CAD build for the part. Positions are in the model's coordinates, mm. Face numbers are marked on the shaded views. A direction names the side the tool comes from. Round coordinates to 2 decimals unless told otherwise and drop trailing zeros. Loops run counter-clockwise (first coordinate to the right, second up) from the corner with the lowest first, then second, coordinate; pieces in that order, holes last.
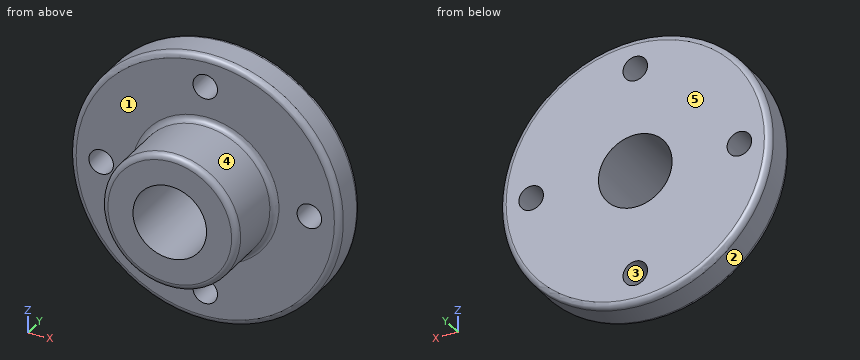
```python
from build123d import *

# Parameters (mm, degrees)
F2_R            = 3.048
F3_R            = 6.35
F4_DEPTH        = 19.051
F4_COPIES_COUNT = 4


# Not quite as in the source:
# - a pattern or mirror of a feature is missing from the dataset's text; its kind, count and spacing are read off the source's solid


with BuildPart() as f1:
    # F0 (on Right) → F1 (revolve)
    with BuildSketch(Plane.YZ):
        Polygon((-53.848, 19.05), (0, 19.05), (0, 69.85), (-19.05, 69.85), (-19.05, 35.052), (-53.848, 35.052), align=None)
    revolve(axis=Axis((0, -30.1634762436, 0), (0, -1, 0)))

    # F2
    f2_edges = [f1.edges().sort_by_distance(p)[0] for p in [
        (0, -53.848, -35.052),
        (0, -19.05, -35.052),
        (0, -19.05, -69.85),
        (0, 0, -69.85),
    ]]
    fillet(f2_edges, radius=F2_R)

    # F3 (on face) → F4 (cut, through all)
    with BuildSketch(Plane.XZ.offset(19.05)):
        with Locations((0, 53.848)):
            Circle(F3_R)
    f4 = extrude(amount=-F4_DEPTH, mode=Mode.SUBTRACT)

    # F4_copies: F4 ×4 about axis
    f4_copies_axis = Axis((0, 0, 0), (0, 1, 0))
    for i in range(1, F4_COPIES_COUNT):
        add(f4.rotate(f4_copies_axis, i * 360 / F4_COPIES_COUNT), mode=Mode.SUBTRACT)


solid = f1.part
```
Item 1: Flat gauge pins, fed straight in: P1, Ø4, axis at x = -24, y = -42.5, coming from the +Z side; P2, Ø6, axis at x = 13.5, y = -29, coming from the -Z side; P3, Ø14.5, axis at x = 0, z = -53.848, coming from the -Y side. Where does each tip first touch, or does it go through?
Answers follow:
P1: stops at z = 27.29
P2: stops at z = -33.44
P3: stops at y = -19.05
Item 2: Cut at D-D, the plane y = -9. Give the cut face in (x, z), plus the area to 3 significant figures.
Answers follow:
outline: circle Ø139.7 at (0, 0); hole circle Ø12.7 at (-53.85, 0); hole circle Ø38.1 at (0, 0); hole circle Ø12.7 at (0, -53.85); hole circle Ø12.7 at (0, 53.85); hole circle Ø12.7 at (53.85, 0)
area: 13,700 mm2
Item 3: Cut at C-C, the plane y = -34.5. Give the cut face in (x, z).
Answers follow:
outline: circle Ø70.1 at (0, 0); hole circle Ø38.1 at (0, 0)
Item 4: 3-axis set-ups, long thin cutter, end or side, ignore diameter. For the marked faces 1 and 2: which of +Z, -Z, +X, -X, +Y, -Y reach the whole face in a straight line?
Answers follow:
face 1: -Y
face 2: +Y, -Y
Item 5: Two-plate mould, pull along Z, no slides. Class the marked faces 3, 4 and 5: released by +Z, released by -Z, zero draft, split by the parting line, or undercut.
Answers follow:
face 3: undercut
face 4: split by the parting line
face 5: zero draft
Item 6: Probe line 1 (Z direction, x = 0, y = -7); line 2 (X direction, y = -34.5, z = 0). List the from-to ranges inside material, lowest first.
Answers follow:
line 1: z = -69.85 to -60.2, -47.5 to -19.05, 19.05 to 47.5, 60.2 to 69.85
line 2: x = -35.05 to -19.05, 19.05 to 35.05
Item 7: Cut at B-B, the plane z = 0. Give the cut face in (x, y), plus the area to 3 significant figures.
Answers follow:
outline: (-69.85, -16) arc R3.05 ccw to (-66.8, -19.05) - (-60.2, -19.05) - (-60.2, 0) - (-66.8, 0) arc R3.05 ccw to (-69.85, -3.05) - close; (-47.5, -19.05) - (-38.1, -19.05) arc R3.05 cw to (-35.05, -22.1) - (-35.05, -50.8) arc R3.05 ccw to (-32, -53.85) - (-19.05, -53.85) - (-19.05, 0) - (-47.5, 0) - close; (19.05, -53.85) - (32, -53.85) arc R3.05 ccw to (35.05, -50.8) - (35.05, -22.1) arc R3.05 cw to (38.1, -19.05) - (47.5, -19.05) - (47.5, 0) - (19.05, 0) - close; (60.2, -19.05) - (66.8, -19.05) arc R3.05 ccw to (69.85, -16) - (69.85, -3.05) arc R3.05 ccw to (66.8, 0) - (60.2, 0) - close
area: 2,560 mm2
Item 8: Cut at A-A, the plane x = 0. Give the cut face in (y, z).
Answers follow:
outline: (-53.85, -32) arc R3.05 ccw to (-50.8, -35.05) - (-22.1, -35.05) arc R3.05 cw to (-19.05, -38.1) - (-19.05, -47.5) - (0, -47.5) - (0, -19.05) - (-53.85, -19.05) - close; (-53.85, 19.05) - (0, 19.05) - (0, 47.5) - (-19.05, 47.5) - (-19.05, 38.1) arc R3.05 cw to (-22.1, 35.05) - (-50.8, 35.05) arc R3.05 ccw to (-53.85, 32) - close; (-19.05, -66.8) arc R3.05 ccw to (-16, -69.85) - (-3.05, -69.85) arc R3.05 ccw to (0, -66.8) - (0, -60.2) - (-19.05, -60.2) - close; (-19.05, 60.2) - (0, 60.2) - (0, 66.8) arc R3.05 ccw to (-3.05, 69.85) - (-16, 69.85) arc R3.05 ccw to (-19.05, 66.8) - close
